Verification items for the finished model (mm, model axes). A direction names the side the tool comes from. Give positions to 0.01 mm unless a question says otherwise; leave off trailing zeros. Loops run counter-clockwise (first coordinate to the right, second up) from the corner with the lowest first, then second, coordinate; pieces in that order, holes last. Notation, with made-up numbers: (69.25, 8) - (91.25, 8) arc R10 ccw to (91.25, 13) - close; hole circle Ø7 at (68.5, 70.5). An arc over 180 degrees is marked (long way). Put each result on its own line as item: value. Start each with the question number.
```python
from build123d import *

# Parameters (mm, degrees)
F0_R     = 4.1
F1_DEPTH = 4
F2_R     = 8
F2_R_2   = 4
F3_DEPTH = 16
F4_DEPTH = 2


with BuildPart() as f1:
    # F0 (on Right) → F1 (new body)
    with BuildSketch(Plane.YZ):
        with BuildLine():
            Line((65, 10), (0, 10))
            ThreePointArc((0, 10), (-10, 0), (0, -10))
            Line((0, -10), (65, -10))
            ThreePointArc((65, -10), (75, 0), (65, 10))
        make_face()
        Circle(F0_R, mode=Mode.SUBTRACT)
        with Locations((25, 0)):
            Circle(F0_R, mode=Mode.SUBTRACT)
    extrude(amount=F1_DEPTH)

    # F2 (on Right) → F3 (join)
    with BuildSketch(Plane.YZ):
        with Locations((65, 0)):
            Circle(F2_R)
        with Locations((65, 0)):
            Circle(F2_R_2, mode=Mode.SUBTRACT)
        with Locations((65, 0)):
            Circle(F2_R_2)
    extrude(amount=F3_DEPTH)

    # F2 (on Right) → F4 (join)
    with BuildSketch(Plane.YZ):
        with Locations((65, 0)):
            Circle(F2_R_2)
    extrude(amount=-F4_DEPTH)


solid = f1.part
```
1) Section check A-A, the plane z = 0. Enter the section's corners in (x, y), plus the area to 3 significant figures.
2) Set-up check for faces 4 (the face through (2, -10, 0)), 5 (the face through (9.916, 58.651, -4.868)): record each of +Z, -Z, +X, -X, +Y, -Y from which the full face is reachable in a straight line by a thin tool's end or side.
3) Section check B-B, the plane y = 25. Enter the section's corners in (x, z), plus the area to 3 significant figures.
4) Scan lines: line 1 along Z through (x, y) = (1.6, 25); line 2 along Y through (x, z) = (1.5, -0.5); line 3 along X through (y, z) = (15, -8). Record each from-to range of solid material in increasing order. Write a range as from..to.
5) Depth check by flat-ended pin: P1, Ø1.5, axis at y = 8, z = 0.5, coming from the -X side; P2, Ø10, axis at y = 15, z = -8, coming from the +X side; P3, Ø6, axis at x = 12, z = 1, coming from the +Y side. Enter the tip coordinate at first touch or a pass-through.
6) Section check C-C, the plane x = 5. Enter the section's corners in (y, z).
7) Section check D-D, the plane y = 43. Enter the section's corners in (x, z).
8) Draft check along Y on faces 1 (the face through (-2, 65, 0)), 2 (the face through (1.972, -0.534, 4.065)), 3 (the face through (-0.986, 68.695, -1.532)). Enter one of: pulls with the +Y half, pulls with the -Y half, needs draft (parallel to the pull), parting line crosses it, or undercut.
Results are:
1. outline: (-2, 61) - (0, 61) - (0, 29.1) - (4, 29.1) - (4, 57) - (16, 57) - (16, 73) - (4, 73) - (4, 75) - (0, 75) - (0, 69) - (-2, 69) - close; (0, -10) - (4, -10) - (4, -4.1) - (0, -4.1) - close; (0, 4.1) - (4, 4.1) - (4, 20.9) - (0, 20.9) - close
1. area: 482 mm2
2. face 4: +X, -X, -Y
2. face 5: +X
3. outline: (0, -10) - (4, -10) - (4, -4.1) - (0, -4.1) - close; (0, 4.1) - (4, 4.1) - (4, 10) - (0, 10) - close
3. area: 47.2 mm2
4. line 1: z = -10..-4.1, 4.1..10
4. line 2: y = -9.99..-4.07, 4.07..20.93, 29.07..74.99
4. line 3: x = 0..4
5. P1: stops at x = 0
5. P2: stops at x = 4
5. P3: stops at y = 73
6. outline: circle Ø16 at (65, 0)
7. outline: (0, -10) - (4, -10) - (4, 10) - (0, 10) - close
8. face 1: needs draft
8. face 2: undercut
8. face 3: parting line crosses it
